Check sheet for the modelled part. Datum: model origin and axes. Units: mm. A direction names the side the tool comes from. Round coordinates to 2 decimals unless told otherwise and drop trailing zeros. Loops run counter-clockwise (first coordinate to the right, second up) from the corner with the lowest first, then second, coordinate; pieces in that order, holes last. Notation, with made-up numbers: (89, -30.75) -> (122, -30.75) arc R24 ccw to (122, -13.75) -> close; hole circle Ø4 at (65, 31). An arc over 180 degrees is marked (long way). Use one line per item in the form item = value. Start each with the question number.
(1) Material ranges on probe 1 along Y at (x, z) = (-43, 8.5); probe 2 along Z at (x, y) = (-54, 40); probe 3 along Z at (x, y) = (-64.5, 41.75), recorded low to high. Write a range as [from, to].
(2) Go/stop test with flat-tipped pins: pin 1 (2 mm diameter, centred on x = -42, y = 43, fed in from +Z); pin 2 (2 mm diameter, centred on x = -53, z = 10, fed in from -Y); pin 3 (1 mm diameter, centred on x = -45.5, z = 11, fed in from +Y); pin 4 (4 mm diameter, centred on y = 33.5, z = 2, fed in from -X). Record where each tip stops, or that it passes through.
(3) Sectioned sample at A-A (z = 11.5). Record the cut outline in (x, y), and give its area (3 significant figures).
(4) Set-up check for faces 4 (the cylindrical face through (-70.23, 39.44, 6.81)), 5 (the cylindrical face through (-43.668, 31.837, 6.81)), 6 (the flat face through (-53, 39, 7)), 7 (the cylindrical face through (-43.67, 46.72, 6.81)): record each of +Z, -Z, +X, -X, +Y, -Y from which the full face is reachable in a straight line by a thin tool's end or side.
(5) Draft check along X on faces 1 (the flat face through (-53, 39, 0)), 2 (the cylindrical face through (-61.8, 46.72, 6.81)), 3 (the cylindrical face through (-47.19, 37, 11.48)). Enter one of: released by +X, released by -X, zero draft, split by the parting line, or undercut.
from build123d import *

# Parameters (mm, degrees)
F1_DEPTH = 10
F2_R     = 6
F3_DEPTH = 3
F5_DEPTH = 6
F6_R     = 0.3
F7_R     = 4


with BuildPart() as f1:
    # F0 (on Top) → F1 (new body)
    with BuildSketch(Plane.XY):
        with BuildLine():
            add(Edge.make_bspline(
                [(-62.732838, 46.778165), (-62.079037, 46.698432), (-61.471616, 46.623094), (-60.905515, 46.552152)],
                knots=[0, 0, 0, 0, 1.102453, 1.102453, 1.102453, 1.102453], degree=3))
            ThreePointArc((-62.732838, 46.778165), (-70.232838, 39.278165), (-62.732838, 31.778165))
            add(Edge.make_bspline(
                [(-62.732838, 31.778165), (-62.096927, 31.853706), (-61.504893, 31.925197), (-60.952079, 31.992638)],
                knots=[0, 0, 0, 0, 1.072287, 1.072287, 1.072287, 1.072287], degree=3))
            ThreePointArc((-60.952079, 31.992638), (-56.833444, 34.647057), (-55.232838, 39.278165))
            ThreePointArc((-55.232838, 39.278165), (-56.818663, 43.890381), (-60.905515, 46.552152))
        make_face()
        with BuildLine():
            ThreePointArc((-60.905515, 46.552152), (-61.812214, 46.721447), (-62.732838, 46.778165))
            add(Edge.make_bspline(
                [(-62.732838, 46.778165), (-62.079037, 46.698432), (-61.471616, 46.623094), (-60.905515, 46.552152)],
                knots=[0, 0, 0, 0, 1.102453, 1.102453, 1.102453, 1.102453], degree=3))
        make_face()
        with BuildLine():
            add(Edge.make_bspline(
                [(-62.732838, 31.778165), (-62.096927, 31.853706), (-61.504893, 31.925197), (-60.952079, 31.992638)],
                knots=[0, 0, 0, 0, 1.072287, 1.072287, 1.072287, 1.072287], degree=3))
            ThreePointArc((-62.732838, 31.778165), (-61.836024, 31.831976), (-60.952079, 31.992638))
        make_face()
        with BuildLine():
            add(Edge.make_bspline(
                [(-60.905515, 46.552152), (-51.802553, 45.411389), (-53.383665, 45.407059), (-44.61111, 46.539163)],
                knots=[1.102453, 1.102453, 1.102453, 1.102453, 18.830007, 18.830007, 18.830007, 18.830007], degree=3))
            ThreePointArc((-60.905515, 46.552152), (-56.818663, 43.890381), (-55.232838, 39.278165))
            ThreePointArc((-55.232838, 39.278165), (-56.833444, 34.647057), (-60.952079, 31.992638))
            add(Edge.make_bspline(
                [(-60.952079, 31.992638), (-51.78057, 33.111525), (-53.404426, 33.115633), (-44.563286, 32.004963)],
                knots=[1.072287, 1.072287, 1.072287, 1.072287, 18.862152, 18.862152, 18.862152, 18.862152], degree=3))
            ThreePointArc((-44.563286, 32.004963), (-50.232797, 39.253486), (-44.61111, 46.539163))
        make_face()
        with BuildLine():
            add(Edge.make_bspline(
                [(-44.61111, 46.539163), (-44.032134, 46.61388), (-43.408059, 46.693547), (-42.732838, 46.778165)],
                knots=[18.830007, 18.830007, 18.830007, 18.830007, 20, 20, 20, 20], degree=3))
            ThreePointArc((-44.61111, 46.539163), (-50.232797, 39.253486), (-44.563286, 32.004963))
            add(Edge.make_bspline(
                [(-44.563286, 32.004963), (-43.997803, 31.933924), (-43.389508, 31.858324), (-42.732838, 31.778165)],
                knots=[18.862152, 18.862152, 18.862152, 18.862152, 20, 20, 20, 20], degree=3))
            ThreePointArc((-42.732838, 31.778165), (-37.429537, 33.974864), (-35.232838, 39.278165))
            ThreePointArc((-35.232838, 39.278165), (-37.429537, 44.581465), (-42.732838, 46.778165))
        make_face()
        with BuildLine():
            ThreePointArc((-42.732838, 46.778165), (-43.679547, 46.718174), (-44.61111, 46.539163))
            add(Edge.make_bspline(
                [(-44.61111, 46.539163), (-44.032134, 46.61388), (-43.408059, 46.693547), (-42.732838, 46.778165)],
                knots=[18.830007, 18.830007, 18.830007, 18.830007, 20, 20, 20, 20], degree=3))
        make_face()
        with BuildLine():
            add(Edge.make_bspline(
                [(-44.563286, 32.004963), (-43.997803, 31.933924), (-43.389508, 31.858324), (-42.732838, 31.778165)],
                knots=[18.862152, 18.862152, 18.862152, 18.862152, 20, 20, 20, 20], degree=3))
            ThreePointArc((-44.563286, 32.004963), (-43.65506, 31.83508), (-42.732838, 31.778165))
        make_face()
    extrude(amount=F1_DEPTH)

    # F2 (on face) → F3 (join)
    with BuildSketch(Plane.XY.offset(10)):
        with Locations((-52.7328, 39.302151)):
            Circle(F2_R)
    extrude(amount=F3_DEPTH)

    # F4 (on face) → F5 (cut)
    with BuildSketch(Plane.XY.offset(13)):
        with BuildLine():
            ThreePointArc((-54.968868, 41.302151), (-53.803266, 36.499634), (-49.7328, 39.302151))
            ThreePointArc((-49.7328, 39.302151), (-49.930283, 40.372617), (-50.496732, 41.302151))
            Line((-50.496732, 41.302151), (-54.968868, 41.302151))
        make_face()
    extrude(amount=-F5_DEPTH, mode=Mode.SUBTRACT)

    # F6
    f6_edges = [f1.edges().sort_by_distance(p)[0] for p in [
        (-70.17612, 40.198788, 10),
        (-52.758079, 45.693906, 10),
        (-35.232879, 39.302843, 10),
        (-52.757446, 32.834331, 10),
    ]]
    fillet(f6_edges, radius=F6_R)

    # F7
    f7_edges = [f1.edges().sort_by_distance(p)[0] for p in [
        (-70.17612, 40.198788, 0),
        (-52.758079, 45.693906, 0),
        (-35.232879, 39.302843, 0),
        (-52.757446, 32.834331, 0),
        (-61.836024, 31.831976, 0),
    ]]
    fillet(f7_edges, radius=F7_R)


solid = f1.part
Checks:
q1.probe_1 = [31.78, 46.77]
q1.probe_2 = [0, 7]
q1.probe_3 = [0, 10]
q2.pin_1 = 10
q2.pin_2 = 32.79
q2.pin_3 = through
q2.pin_4 = -68.9
q3.outline = circle Ø12 at (-52.73, 39.3); hole (-54.97, 41.3) arc R3 ccw (long way) to (-49.73, 39.3) arc R3 ccw to (-50.5, 41.3) -> close
q3.area = 87.9 mm2
q4.face_4 = +Z, -Z, -X
q4.face_5 = +Z, -Z, -Y
q4.face_6 = +Z
q4.face_7 = +Z, -Z, +Y
q5.face_1 = zero draft
q5.face_2 = undercut
q5.face_3 = split by the parting line
